For this review, use the dimensioned drawing (mm, ordinates from the lowest corner) and the shaded views. A direction names the side the tool comes from. Round coordinates to 2 decimals unless told otherwise and drop trailing zeros. Loops run counter-clockwise (first coordinate to the right, second up) from the corner with the lowest first, then second, coordinate; pieces in that order, holes last. Notation, with made-up numbers: (65.5, 58.25) - (92.5, 58.25) arc R4 ccw to (92.5, 63.25) - close; hole circle Ø9 at (13.25, 74.25). An arc over 180 degrees is marked (long way). Use one line per item in the form item = value. Start each with the question number.
(1) The part is to be moulded in two halves that separate along Z. For the marked faces 4, 5 and 6, say which applies: released by +Z, released by -Z, zero draft, split by the parting line, or undercut.
(2) Machinability: for the marked faces 1, 2 and 3, which of the approach directions +Z, -Z, +X, -X, +Y, -Y give a long, thin tool a straight path to every point of the face, cutting with its end or side? Answer none if there is none.
(3) We need section B-B, the plane x = 10. Write out the cut boundary in (y, z), then the cut area to 3 significant figures.
(4) For pin 1 (5 mm diameter, centred on y = 6, z = 10, fed in from -X); pin 2 (5 mm diameter, centred on x = 9, z = 10.5, fed in from +Y); pin 3 (5 mm diameter, centred on y = 5, z = 12.5, fed in from +X), all flat-tipped, find the tip position at first contact; note any pin that passes through.
(5) We need section C-C, the plane y = 27. Write out the cut boundary in (x, z).
(6) We need section D-D, the plane x = 1.5. Write out the cut boundary in (y, z), then the cut area to 3 significant figures.
(7) Wall thickness on probe 1 along Z at (x, y) = (8.75, 25.5); probe 2 along Y at (x, z) = (10, 18.65); probe 3 along Y at (x, z) = (16.5, 15): over which ranges is each line inside the solid? List them lowest first. Write a range as [from, to].
(8) We need section A-A, the plane z = 19. Write out the cut boundary in (x, y) (1 decimal), then the cut area to 3 significant figures.
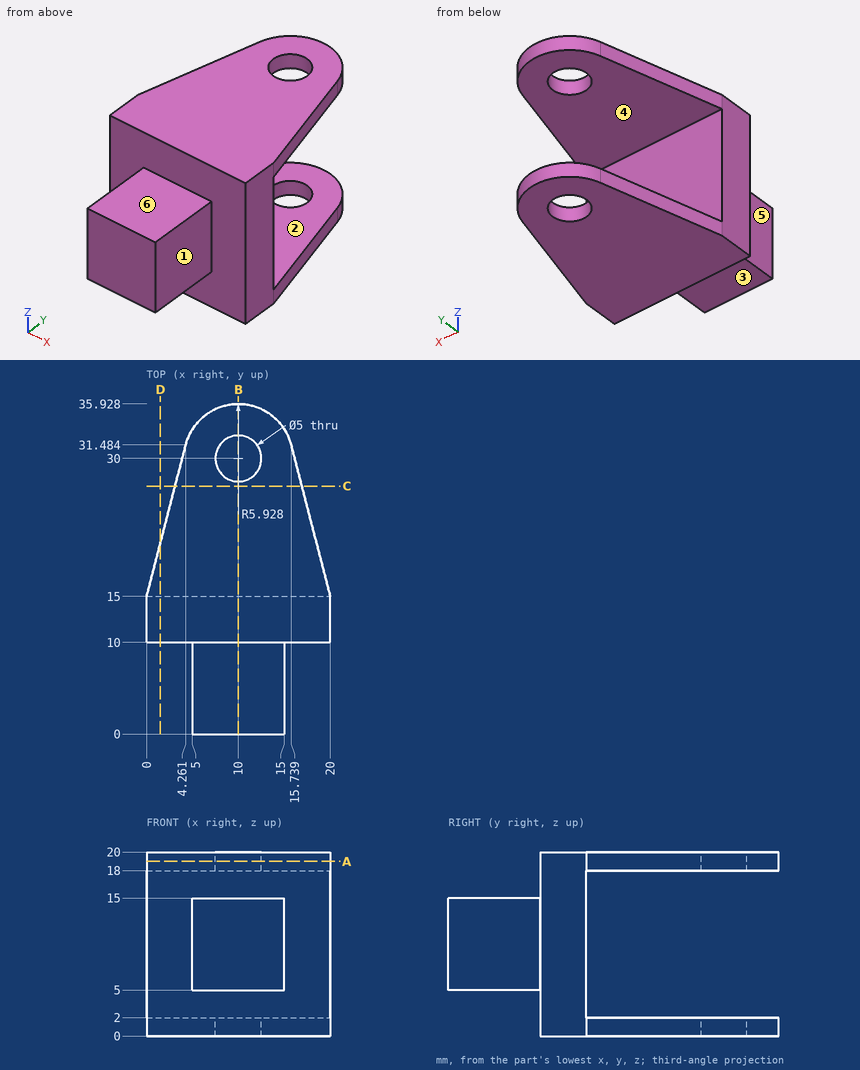
Data:
q1.face_4 = undercut
q1.face_5 = zero draft
q1.face_6 = released by +Z
q2.face_1 = +Z, -Z, +X, -Y
q2.face_2 = +X, -X, +Y
q2.face_3 = -Z, +X, -X, -Y
q3.outline = (0, 5) - (10, 5) - (10, 0) - (27.5, 0) - (27.5, 2) - (15, 2) - (15, 18) - (27.5, 18) - (27.5, 20) - (10, 20) - (10, 15) - (0, 15) - close; (32.5, 0) - (35.93, 0) - (35.93, 2) - (32.5, 2) - close; (32.5, 18) - (35.93, 18) - (35.93, 20) - (32.5, 20) - close
q3.area = 264 mm^2
q4.pin_1 = 5
q4.pin_2 = 15
q4.pin_3 = 15
q5.outline = (3.1, 0) - (16.9, 0) - (16.9, 2) - (3.1, 2) - close; (3.1, 18) - (16.9, 18) - (16.9, 20) - (3.1, 20) - close
q6.outline = (10, 0) - (20.8, 0) - (20.8, 2) - (15, 2) - (15, 18) - (20.8, 18) - (20.8, 20) - (10, 20) - close
q6.area = 123 mm^2
q7.probe_1 = [0, 2], [18, 20]
q7.probe_2 = [10, 27.5], [32.5, 35.93]
q7.probe_3 = [10, 15]
q8.outline = (0, 10) - (20, 10) - (20, 15) - (15.7, 31.5) arc R5.9 ccw to (4.3, 31.5) - (0, 15) - close; hole circle Ø5 at (10, 30)
q8.area = 378 mm^2
